Geometry: final body of the model. Coordinates: model frame, mm. Face numbers are marked on the shaded views. Round coordinates to 2 decimals unless told otherwise and drop trailing zeros. Loops run counter-clockwise (first coordinate to the right, second up) from the corner with the lowest first, then second, coordinate; pieces in that order, holes last. Notation, with made-up numbers: M 49,14 L 81,14 A4 cw 81,21 Z; hole C 34.5,-35 d8. An arc over 180 degrees is marked long. Return JSON: item names as keys, results as strings.
from build123d import *

# Parameters (mm, degrees)
SKETCH2_R           = 27.5
SKETCH2_R_2         = 15
BOSS_EXTRUDE1_DEPTH = 110
SKETCH3_R           = 27.5
SKETCH3_R_2         = 15
BOSS_EXTRUDE2_DEPTH = 55


with BuildPart() as part:
    # Sketch2 → Boss-Extrude1 (new body)
    with BuildSketch(Plane(origin=(0, 0, 0), x_dir=(1, 0, 0), z_dir=(0, 1, 0))):
        with Locations(Location((0, 0, 0), (0, 0, 270))):
            Circle(SKETCH2_R)
        with Locations(Location((0, 0, 0), (0, 0, 270))):
            Circle(SKETCH2_R_2, mode=Mode.SUBTRACT)
    extrude(amount=BOSS_EXTRUDE1_DEPTH)

    # Sketch3 → Boss-Extrude2 (add, symmetric)
    with BuildSketch(Plane.XY):
        with Locations((38, 55)):
            Circle(SKETCH3_R)
        with Locations((38, 55)):
            Circle(SKETCH3_R_2, mode=Mode.SUBTRACT)
    extrude(amount=BOSS_EXTRUDE2_DEPTH, both=True)


solid = part.part
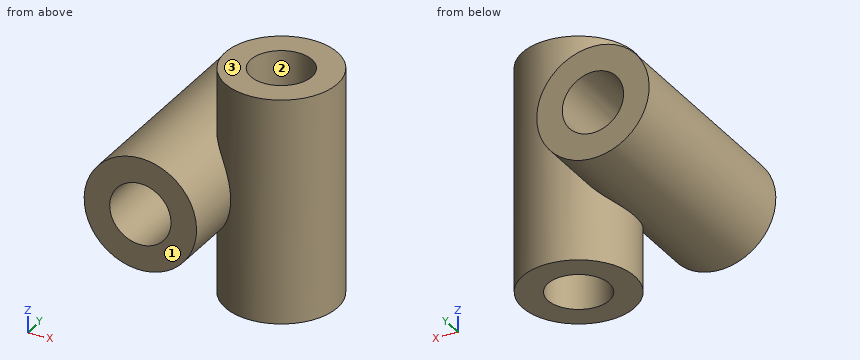
Q1. Section query D-D (y = 73.5). Output: boundary loops of the cut face in (x, z).
Determined:
{"outline": "M 17.65,-55 L 58.35,-55 L 58.35,55 L 17.65,55 L 17.65,21.09 A27.5 ccw long 17.65,-21.09 Z; hole C 0,0 d30"}
Q2. Pin query (flat end, axial travel): pin 1 (8 mm diameter, centred on x = 32.5, z = -15.5, fed in from +Y); pin 2 (12 mm diameter, centred on y = 11.5, z = -31.5, fed in from +X); pin 3 (5 mm diameter, centred on x = 1.5, y = 45.5, fed in from +Z). Return the tip coordinate at first contact, or that it passes through.
Determined:
{"pin 1": "stops at y = 82.46", "pin 2": "stops at x = 10.3", "pin 3": "stops at z = 27.5"}
Q3. Material intervals for L1, parallel to Z at x = 0.5, y = 38.5; L2, parallel to Y at x = 38, z = 24.5; L3, parallel to Y at x = 42.5, z = 17, sorted ascending.
Determined:
{"L1": "z = -27.5 to -14.99, 14.99 to 27.5", "L2": "y = 27.5 to 40, 70 to 82.5", "L3": "y = 27.87 to 40.69, 69.31 to 82.13"}
Q4. Pull-direction query (Y, two-part tool) for the marked faces 1, 2 and 3; classes: pulls with the +Y half, pulls with the -Y half, needs draft (parallel to the pull), parting line crosses it, or undercut.
Determined:
{"face 1": "pulls with the -Y half", "face 2": "undercut", "face 3": "needs draft"}
Q5. Section query A-A (z = 0). Output: boundary loops of the cut face in (x, y).
Determined:
{"outline": "M -27.5,0 L -15,0 L -15,110 L -27.5,110 Z; M 15,0 L 27.5,0 L 27.5,29.58 A27.5 ccw long 27.5,80.42 L 27.5,110 L 15,110 L 15,70.07 A27.5 ccw 15,39.93 Z; hole M 27.5,44.29 A15 ccw long 27.5,65.71 Z"}
Q6. Section query C-C (y = 52). Output: boundary loops of the cut face in (x, z), plus the area to 3 significant figures.
Determined:
{"outline": "M 10.66,-55 L 23.3,-55 L 23.3,-14.6 A27.5 ccw 23.3,14.6 L 23.3,55 L 10.66,55 L 10.66,25.35 A27.5 ccw long 10.66,-25.35 Z; M 52.7,-55 L 65.34,-55 L 65.34,55 L 52.7,55 Z; hole M 10.66,-10.55 L 10.66,10.55 A15 ccw long Z", "area": "3,980 mm^2"}
Q7. Section query B-B (x = 38). Output: boundary loops of the cut face in (y, z), plus the area to 3 significant figures.
Determined:
{"outline": "M 27.5,-55 L 40,-55 L 40,55 L 27.5,55 Z; M 70,-55 L 82.5,-55 L 82.5,55 L 70,55 Z", "area": "2,750 mm^2"}
